from build123d import *

# Parameters (mm, degrees)
SKETCH1_R           = 30
BOSS_EXTRUDE1_DEPTH = 10


with BuildPart() as part:
    # Sketch1 → Boss-Extrude1 (new body)
    with BuildSketch(Plane(origin=(0, 0, 0), x_dir=(1, 0, 0), z_dir=(0, 1, 0))):
        with BuildLine():
            Line((-21.391856852, 38.422206609), (-50.810091155, 146.458168919))
            Line((-50.810091155, 146.458168919), (-8.048011127, 280.566292355))
            Line((-8.048011127, 280.566292355), (0, 392.18316322))
            Line((0, 392.18316322), (8.048011127, 280.566292355))
            Line((8.048011127, 280.566292355), (50.810091155, 146.458168919))
            Line((50.810091155, 146.458168919), (21.391856852, 38.422206609))
            ThreePointArc((21.391856852, 38.422206609), (0, -43.97587407), (-21.391856852, 38.422206609))
        make_face()
        Circle(SKETCH1_R, mode=Mode.SUBTRACT)
        Polygon((0, 238.738180914), (-21.391856852, 146.458168919), (0, 60.077729237), (21.391856852, 146.458168919), align=None, mode=Mode.SUBTRACT)
    extrude(amount=BOSS_EXTRUDE1_DEPTH)


solid = part.part
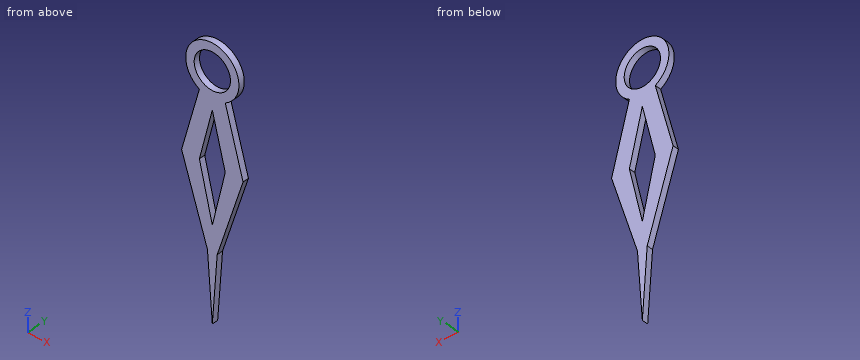
Work out the finished part from the listing and answer in its coordinate system (mm). Coordinates: 2 decimals unless noted, no trailing zeros. Loops run counter-clockwise (first coordinate to the right, second up) from the corner with the lowest first, then second, coordinate; pieces in that order, holes last. Notation, with made-up numbers: (85, 32.25) -> (94, 32.25) arc R30 ccw to (94, 63.25) -> close; hole circle Ø11 at (2, 7). An arc over 180 degrees is marked (long way). Answer as CSV lines item,"result".
1) Flat-ended cylindrical pins translate along their axes: pin 1 (1 mm diameter, centred on y = 8, z = -294.5, fed in from +X); pin 2 (4 mm diameter, centred on y = 9, z = -136, fed in from +X); pin 3 (3 mm diameter, centred on y = 7.5, z = -137.5, fed in from +X). Find the tip coordinate at first contact, or state that the pin passes through.
A:
pin 1,"stops at x = 7.08"
pin 2,"stops at x = 48.51"
pin 3,"stops at x = 48.78"
2) Straight lines are drawn through the part: probe 1 along X at (y, z) = (2.75, 0); probe 2 along X at (y, z) = (2.25, -190); probe 3 along X at (y, z) = (9.5, -263.5). For each, find the intervals that lie inside material, in ascending order.
A:
probe 1,"x = -43.98 to -30, 30 to 43.98"
probe 2,"x = -36.93 to -11.3, 11.3 to 36.93"
probe 3,"x = -13.49 to 13.49"
3) The part is cut by section B-B (x = -38.5). Give the vertices of the cut face in (y, z).
A:
outline,"(0, -185.06) -> (10, -185.06) -> (10, -101.25) -> (0, -101.25) -> close; (0, -21.25) -> (10, -21.25) -> (10, 21.25) -> (0, 21.25) -> close"
4) The part is cut by section A-A (z = 0). Give the vertices of the cut face in (x, y).
A:
outline,"(-43.98, 0) -> (-30, 0) -> (-30, 10) -> (-43.98, 10) -> close; (30, 0) -> (43.98, 0) -> (43.98, 10) -> (30, 10) -> close"
5) The part is cut by section C-C (y = 7.5). Give the vertices of the cut face in (x, z), and give its area (3 significant figures).
A:
outline,"(-50.81, -146.46) -> (-8.05, -280.57) -> (0, -392.18) -> (8.05, -280.57) -> (50.81, -146.46) -> (21.39, -38.42) arc R43.98 ccw (long way) to (-21.39, -38.42) -> close; hole circle Ø60 at (0, 0); hole (-21.39, -146.46) -> (0, -238.74) -> (21.39, -146.46) -> (0, -60.08) -> close"
area,"15,900 mm²"
